from build123d import *

# Parameters (mm, degrees)
SKETCH1_R           = 4
BOSS_EXTRUDE1_DEPTH = 25
SKETCH2_W           = 25.15
SKETCH2_H           = 5
CUT_EXTRUDE1_DEPTH  = 20


with BuildPart() as part:
    # Sketch1 → Boss-Extrude1 (new body)
    with BuildSketch(Plane(origin=(0, 0, 0), x_dir=(1, 0, 0), z_dir=(0, 1, 0))):
        with BuildLine():
            Line((0, 0), (35.106623938, 0))
            ThreePointArc((35.106623938, 0), (39.654705316, 1.418590137), (42.589820847, 5.171261055))
            Line((42.589820847, 5.171261055), (63.093196909, 59.411261055))
            ThreePointArc((63.093196909, 59.411261055), (58.438738945, 69.723196909), (48.126803091, 65.068738945))
            Line((48.126803091, 65.068738945), (30.799975774, 19.232038159))
            ThreePointArc((30.799975774, 19.232038159), (28.965528567, 16.886618836), (26.122977706, 16))
            Line((26.122977706, 16), (0, 16))
            ThreePointArc((0, 16), (-8, 8), (0, 0))
        make_face()
        with Locations(Location((0, 8, 0), (0, 0, 270))):
            Circle(SKETCH1_R, mode=Mode.SUBTRACT)
        with Locations(Location((55.61, 62.24, 0), (0, 0, 270))):
            Circle(SKETCH1_R, mode=Mode.SUBTRACT)
        with Locations(Location((34.72, 8, 0), (0, 0, 270))):
            Circle(SKETCH1_R, mode=Mode.SUBTRACT)
    extrude(amount=BOSS_EXTRUDE1_DEPTH)

    # Sketch2 → Cut-Extrude1 (cut)
    with BuildSketch(Plane.XY):
        with Locations((4.575, 12.5)):
            Rectangle(SKETCH2_W, SKETCH2_H)
    extrude(amount=-CUT_EXTRUDE1_DEPTH, mode=Mode.SUBTRACT)


solid = part.part
The model under review builds one solid part; all positions refer to its coordinate system, in mm. A direction names the side the tool comes from. Round coordinates to 2 decimals unless told otherwise and drop trailing zeros. Loops run counter-clockwise (first coordinate to the right, second up) from the corner with the lowest first, then second, coordinate; pieces in that order, holes last. Notation, with made-up numbers: (-32, 87.25) -> (6, 87.25) arc R11 ccw to (6, 104.25) -> close; hole circle Ø7 at (5.5, 16). An arc over 180 degrees is marked (long way). Answer as CSV lines item,"result".
1) To check wall thickness, follow line 1 along X through (y, z) = (22, -7.5); line 2 along Y through (x, z) = (16, -11.5); line 3 along Z through (x, y) = (0, 5.75). State the ranges of each line that lie inside material, in increasing order. Write a range as from..to.
Geometry results:
line 1,"x = -7.98..-3.97, 3.97..30.75, 38.69..43.47"
line 2,"y = 0..10, 15..25"
line 3,"z = -16..-12, -4..0"
2) For P1, Ø1, axis at x = 3, y = 11, coming from the -Z side; P2, Ø1, axis at y = 11, z = -43.5, coming from the -X side; P3, Ø2.5, axis at y = 12, z = -6.5, coming from the -X side; P4, Ø1, axis at y = 19.5, z = -10.5, coming from the +X side, all flat-tipped, find the tip position at first contact; note any pin that passes through.
Geometry results:
P1,"passes through"
P2,"stops at x = 39.78"
P3,"stops at x = 17.15"
P4,"stops at x = 44.79"
3) Tool access review of faces 1 (the face through (7, 15, -8)), 2 (the face through (-2.4, 19.9, -11.2)): name each direction out of +Z, -Z, +X, -X, +Y, -Y from which nothing blocks a thin tool from reaching the whole face with its end or side.
Geometry results:
face 1,"+Z, -Z, -X"
face 2,"+Y, -Y"
4) Add section A-A on x = 15. Write out the cut boundary in (y, z).
Geometry results:
outline,"(0, -16) -> (10, -16) -> (10, 0) -> (0, 0) -> close; (15, -16) -> (25, -16) -> (25, 0) -> (15, 0) -> close"
5) Add section D-D on x = 1. Write out the cut boundary in (y, z).
Geometry results:
outline,"(0, -16) -> (10, -16) -> (10, -11.87) -> (0, -11.87) -> close; (0, -4.13) -> (10, -4.13) -> (10, 0) -> (0, 0) -> close; (15, -16) -> (25, -16) -> (25, -11.87) -> (15, -11.87) -> close; (15, -4.13) -> (25, -4.13) -> (25, 0) -> (15, 0) -> close"
6) Add section C-C on z = -62.24. Write out the cut boundary in (x, y), plus the area to 3 significant figures.
Geometry results:
outline,"(47.06, 0) -> (51.61, 0) -> (51.61, 25) -> (47.06, 25) -> close; (59.61, 0) -> (63.61, 0) -> (63.61, 25) -> (59.61, 25) -> close"
area,"214 mm²"
7) Draft analysis for pull direction Z (two halves, no side actions). For faces 3 (the face through (55.786, 12.325, -66.236)), 4 (the face through (13.2, 9.5, -16)), 5 (the face through (-2.4, 4.9, -11.2)), 6 (the face through (-8, 5, -8)), state which applies: pulls with the +Z half, pulls with the -Z half, needs draft (parallel to the pull), parting line crosses it, or undercut.
Geometry results:
face 3,"undercut"
face 4,"pulls with the -Z half"
face 5,"undercut"
face 6,"parting line crosses it"
8) Add section B-B on z = -8. Write out the cut boundary in (x, y), plus the area to 3 significant figures.
Geometry results:
outline,"(-8, 0) -> (-4, 0) -> (-4, 10) -> (-8, 10) -> close; (-8, 15) -> (-4, 15) -> (-4, 25) -> (-8, 25) -> close; (4, 0) -> (30.72, 0) -> (30.72, 25) -> (4, 25) -> (4, 15) -> (17.15, 15) -> (17.15, 10) -> (4, 10) -> close; (38.72, 0) -> (43.66, 0) -> (43.66, 25) -> (38.72, 25) -> close"
area,"806 mm²"
